The model under review builds one solid part; all positions refer to its coordinate system, in mm. Face numbers are marked on the shaded views. Give positions to 0.01 mm unless a question says otherwise; leave off trailing zeros. Write each loop counter-clockwise with the first axis right and the second up, starting at its lowest first coordinate (ties: lowest second). Pieces come first, ordered by that corner, then holes.
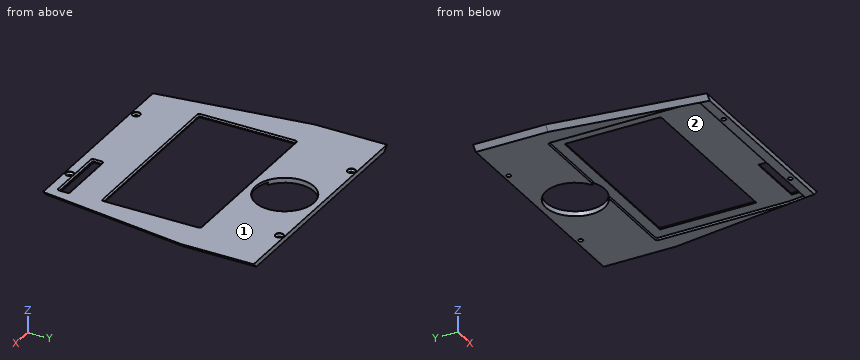
from build123d import *

# Parameters (mm, degrees)
SKETCH1_R                                    = 40
SKETCH1_W                                    = 120
SKETCH1_H                                    = 18.5
SKETCH1_W_2                                  = 344.2
SKETCH1_H_2                                  = 193.6
BOSS_EXTRUDE1_DEPTH                          = 5
CUT_EXTRUDE1_DEPTH                           = 5
SKETCH3_R                                    = 59
CUT_EXTRUDE2_DEPTH                           = 491.321307177
FILLET1_R                                    = 1
FILLET2_R                                    = 2
CHAMFER1_SIZE                                = 3
CHAMFER2_SIZE                                = 10
CSK_FOR_M8_HEX_SOCKET_COUNTERSUNK_HE_2_COUNT = 2
CSK_FOR_M8_HEX_SOCKET_COUNTERSUNK_HE_2_PITCH = 260
CSK_FOR_M8_HEX_SOCKET_COUNTERSUNK_HE_3_COUNT = 2
CSK_FOR_M8_HEX_SOCKET_COUNTERSUNK_HE_3_PITCH = 494.801980594
CSK_FOR_M8_HEX_SOCKET_COUNTERSUNK_HE_4_COUNT = 2
CSK_FOR_M8_HEX_SOCKET_COUNTERSUNK_HE_4_PITCH = 427.117079968
FILLET3_R                                    = 5


with BuildPart() as part:
    # Sketch1 → Boss-Extrude1 (new, symmetric)
    with BuildSketch(Plane.XY.offset(5)):
        Polygon((-198.5, -20), (198.5, -20), (240.802791245, 281), (240.802791245, 427), (-240.802791245, 427), (-240.802791245, 281), align=None)
        with Locations((0, 355.5)):
            Circle(SKETCH1_R, mode=Mode.SUBTRACT)
        with Locations((117.5, 10.25)):
            Rectangle(SKETCH1_W, SKETCH1_H, mode=Mode.SUBTRACT)
        with Locations((0, 184.15)):
            Rectangle(SKETCH1_W_2, SKETCH1_H_2, mode=Mode.SUBTRACT)
    extrude(amount=BOSS_EXTRUDE1_DEPTH, both=True)

    # Sketch2 → Cut-Extrude1 (cut)
    with BuildSketch(Plane(origin=(0, 0, 0), x_dir=(-1, 0, 0), z_dir=(0, 0, -1))):
        with BuildLine():
            Line((196, 34.064541037), (196, 68.5))
            Line((196, 68.5), (196, 297))
            ThreePointArc((196, 297), (194.535533906, 300.535533906), (191, 302))
            Line((191, 302), (-191, 302))
            ThreePointArc((-191, 302), (-194.535533906, 300.535533906), (-196, 297))
            Line((-196, 297), (-196, 68.5))
            Line((-196, 68.5), (-196, 34.064541037))
            Line((-196, 34.064541037), (-191.072000134, -1))
            Line((-191.072000134, -1), (191.072000134, -1))
            Line((191.072000134, -1), (196, 34.064541037))
        make_face()
    extrude(amount=-CUT_EXTRUDE1_DEPTH, mode=Mode.SUBTRACT)

    # Sketch3 → Cut-Extrude2 (cut, through all)
    with BuildSketch(Plane.XY.offset(10)):
        with Locations((0, 355.5)):
            Circle(SKETCH3_R)
    extrude(amount=-CUT_EXTRUDE2_DEPTH, mode=Mode.SUBTRACT)

    # Fillet1
    fillet1_edges = [part.edges().sort_by_distance(p)[0] for p in [
        (177.5, 1, 7.5),
        (177.5, 19.5, 7.5),
        (57.5, 19.5, 7.5),
        (57.5, 1, 7.5),
        (-172.1, 280.95, 7.5),
        (-172.1, 87.35, 7.5),
        (172.1, 87.35, 7.5),
        (172.1, 280.95, 7.5),
    ]]
    fillet(fillet1_edges, radius=FILLET1_R)

    # Fillet2
    fillet2_edges = [part.edges().sort_by_distance(p)[0] for p in [
        (-24.874685928, 302, 2.5),
        (24.874685928, 302, 2.5),
    ]]
    fillet(fillet2_edges, radius=FILLET2_R)

    # Chamfer1
    chamfer1_edges = [part.edges().sort_by_distance(p)[0] for p in [
        (57.5, 10.25, 10),
        (117.5, 1, 10),
        (117.5, 19.5, 10),
        (177.5, 10.25, 10),
        (0, 87.35, 10),
        (172.1, 184.15, 10),
        (0, 280.95, 10),
        (-172.1, 184.15, 10),
        (57.792893219, 1.292893219, 10),
        (57.792893219, 19.207106781, 10),
        (177.207106781, 19.207106781, 10),
        (177.207106781, 1.292893219, 10),
        (171.807106781, 87.642893219, 10),
        (171.807106781, 280.657106781, 10),
        (-171.807106781, 280.657106781, 10),
        (-171.807106781, 87.642893219, 10),
    ]]
    chamfer(chamfer1_edges, length=CHAMFER1_SIZE)

    # Chamfer2
    chamfer2_edges = [part.edges().sort_by_distance(p)[0] for p in [
        (219.651395623, 130.5, 0),
        (240.802791245, 354, 0),
        (-219.651395623, 130.5, 0),
        (-240.802791245, 354, 0),
    ]]
    chamfer(chamfer2_edges, length=CHAMFER2_SIZE - 0.0001)  # a hair under: the kernel refuses the full size

    # Sketch5 → CSK for M8 Hex Socket Countersunk Head Screw1 (revolve, cut)
    with BuildSketch(Plane(origin=(-130, 417, 10), x_dir=(0, -1, 0), z_dir=(1, 0, 0))):
        Polygon((0, 0), (0, 10), (4.5, 10), (4.5, 4.5), (8, 1), (8, 0), align=None)
    csk_for_m8_hex_socket_countersunk_head_s = revolve(axis=Axis((-130, 417, 16.35), (0, 0, -1)), mode=Mode.SUBTRACT)

    # CSK for M8 Hex Socket Countersunk He 2: CSK for M8 Hex Socket Countersunk Head Screw1 ×2
    with Locations(*[(i * CSK_FOR_M8_HEX_SOCKET_COUNTERSUNK_HE_2_PITCH, 0, 0) for i in range(1, CSK_FOR_M8_HEX_SOCKET_COUNTERSUNK_HE_2_COUNT)]):
        add(csk_for_m8_hex_socket_countersunk_head_s, mode=Mode.SUBTRACT)

    # CSK for M8 Hex Socket Countersunk He 3: CSK for M8 Hex Socket Countersunk Head Screw1 ×2
    with Locations(*[Vector(0.5052526259085499, -0.8629714850518034, 0) * (i * CSK_FOR_M8_HEX_SOCKET_COUNTERSUNK_HE_3_PITCH) for i in range(1, CSK_FOR_M8_HEX_SOCKET_COUNTERSUNK_HE_3_COUNT)]):
        add(csk_for_m8_hex_socket_countersunk_head_s, mode=Mode.SUBTRACT)

    # CSK for M8 Hex Socket Countersunk He 4: CSK for M8 Hex Socket Countersunk Head Screw1 ×2
    with Locations(*[Vector(0.02341278414986336, -0.9997258831991657, 0) * (i * CSK_FOR_M8_HEX_SOCKET_COUNTERSUNK_HE_4_PITCH) for i in range(1, CSK_FOR_M8_HEX_SOCKET_COUNTERSUNK_HE_4_COUNT)]):
        add(csk_for_m8_hex_socket_countersunk_head_s, mode=Mode.SUBTRACT)

    # Fillet3
    fillet3_edges = [part.edges().sort_by_distance(p)[0] for p in [
        (-196, 34.064541037, 2.5),
        (-191.072000134, -1, 2.5),
        (191.072000134, -1, 2.5),
        (196, 34.064541037, 2.5),
    ]]
    fillet(fillet3_edges, radius=FILLET3_R)


solid = part.part
1) The part is to be moulded in two halves that separate along X. For the marked faces 1 and 2, say which applies: +X half, -X half, draft (parallel to the pull), parting line (faces both ways), or undercut.
2) Consider section B-B, the plane z = 1.75. Give the boundary of the cut face in (x, y), then the cut area to 3 significant figures.
3) To check wall thickness, follow probe 1 along Y at (x, z) = (-91.5, 7); probe 2 along Y at (x, z) = (153, 0.5); probe 3 along Y at (x, z) = (130, 9.4). State the ranges of each line that lie inside material, in increasing order.
4) Insertion check: pin 1 (1.5 mm diameter, centred on y = 287, z = 8.5, fed in from +X); pin 2 (0.6 mm diameter, centred on y = 178, z = 6.5, fed in from -X); pin 3 (2 mm diameter, centred on y = 13.5, z = 6, fed in from -X). Each pin has a flat end and moves straight along its axis. Give the tip position at first contact, or say it passes through.
Answer block:
1. face 1: draft
1. face 2: undercut
2. outline: (-232.55, 281.58) - (-190.17, -20) - (190.17, -20) - (232.55, 281.58) - (232.55, 427) - (-232.55, 427) - close; hole (-196, 34.41) arc R5 ccw to (-195.95, 33.72) - (-191.68, 3.3) arc R5 ccw to (-186.73, -1) - (186.73, -1) arc R5 ccw to (191.68, 3.3) - (195.95, 33.72) arc R5 ccw to (196, 34.41) - (196, 297) arc R5 ccw to (191, 302) - (32.69, 302) arc R2 cw to (31.62, 305.69) arc R59 ccw (long way) to (-31.62, 305.69) arc R2 cw to (-32.69, 302) - (-191, 302) arc R5 ccw to (-196, 297) - close; hole circle Ø9 at (-130, 417); hole circle Ø9 at (-120, -10); hole circle Ø9 at (120, -10); hole circle Ø9 at (130, 417)
2. area: 65,500 mm2
3. probe 1: y = -20 to 87.35, 280.95 to 427
3. probe 2: y = -20 to -1, 302 to 427
3. probe 3: y = -20 to -1.4, 21.9 to 84.95, 283.35 to 409, 425 to 427
4. pin 1: stops at x = 240.05
4. pin 2: stops at x = -223.1
4. pin 3: stops at x = -200.19
